Autodesk Inventor part; units mm, degrees
ref_plane "YZ Plane" through (0, 0, 0) normal (1, 0, 0) x (0, 1, 0)
ref_plane "XZ Plane" through (0, 0, 0) normal (0, 1, 0) x (-1, 0, 0)
ref_plane "XY Plane" through (0, 0, 0) normal (0, 0, 1) x (1, 0, 0)
sketch "Sketch1" plane through (0, 0, 0) normal (0, 0, 1) x (1, 0, 0)
  spline S0 degree 3 poles (12.7758, 13.7437) (13.4536, 14.296) (14.1651, 14.793) (16.9373, 16.4418) (19.2243, 17.2436) (24.5957, 17.9791) (27.7237, 17.5963) (32.8694, 15.5351) (34.9647, 14.1297) (38.6283, 10.3594) (40.0896, 7.8966) (41.4354, 3.545) (41.7033, 1.7728) (41.7033, 0) (41.7033, -1.7729) (41.4354, -3.5451) (40.0895, -7.897) (38.6278, -10.3602) (34.9655, -14.1286) (32.8727, -15.5328) (27.7225, -17.598) (24.5861, -17.9808) (19.2198, -17.2406) (16.945, -16.4433) (14.1759, -14.8006) (13.4587, -14.3002) (12.7758, -13.7437) knots 0.047577 0.047577 0.047577 0.047577 0.308418 0.308418 1.015437 1.015437 1.927825 1.927825 2.666741 2.666741 3.497446 3.497446 4.02653 4.02653 4.02653 4.555615 4.555615 5.386442 5.386442 6.124601 6.124601 7.039356 7.039356 7.74266 7.74266 8.00548 8.00548 8.00548 8.00548 weights 1 1 1 1 1 1 1 1 1 1 1 1 1 1 1 1 1 1 1 1 1 1 1 1 1 1 1
  spline S1 degree 3 poles (12.7758, -13.7437) (12.3265, -13.3776) (11.8219, -13.0794) (10.6568, -12.62) (9.9847, -12.4901) (9.3118, -12.4901) knots 0 0 0 0 0.462707 0.462707 1 1 1 1 weights 1 1 1 1 1 1
  line L0 (9.3118, -12.4901) -> (-31.0253, -12.4901)
  spline S2 degree 3 poles (9.3118, 12.4901) (9.7991, 12.4901) (10.2862, 12.5578) (11.492, 12.896) (12.1826, 13.2604) (12.7758, 13.7437) knots 0 0 0 0 0.389114 0.389114 1 1 1 1 weights 1 1 1 1 1 1
  line L1 (0, 0) -> (-42.2873, 0) construction
  line L2 (9.3118, 12.4901) -> (-31.0253, 12.4901)
  arc A0 (-31.0253, 12.4901) -> (-31.0253, -12.4901) centre (-31.0253, 0) ccw
extrude "Extrusion1" add sketch "Sketch1" along normal blind 2.5
chamfer "Chamfer1" distance 2 angle 50 6 edges at (41.7033, 0, 2.5) (11.1518, -12.8172, 2.5) (-10.8568, -12.4901, 2.5) (-43.5155, 0, 2.5) (-10.8568, 12.4901, 2.5) (11.1517, 12.8172, 2.5) measured on face at (-4.1339, -4.1634, 2.5)
sketch "Sketch6" plane through (0, 0, 2.5) normal (0, 0, 1) x (1, 0, 0)
  line L0 (-9.5253, -2.5425) -> (-15.3564, -2.5425) construction
  line L1 (-15.3564, -2.5425) -> (-15.3564, 2.5425) construction
  line L2 (-15.3564, 2.5425) -> (-9.5253, 2.5425) construction
  line L3 (-9.5253, 2.5425) -> (-9.5253, -2.5425) construction
  point P0 (0, 0)
  point P1 (-6.2263, 0)
decal "Decal1"
ref_plane "Work Plane1" through (0, 0, 0) normal (0.2164396, 0, 0.976296) x (0, 1, 0)
sketch "Sketch7" plane through (0, 0, 0) normal (0.2164396, 0, 0.976296) x (0, 1, 0)
  point P0 (0, 0)
ref_plane "Work Plane2" through (0, 0, 0) normal (0.2164396, 0, 0.976296) x (0, 1, 0)
properties part number "gornji shiny dio"
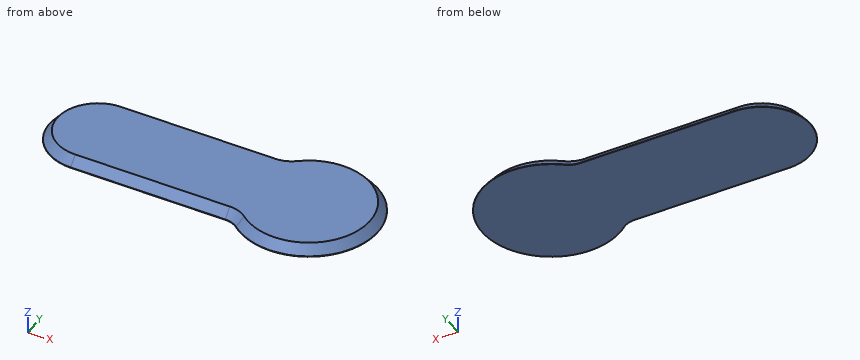
For this review, take the finished solid that the model builds, in its own axes (mm). Round coordinates to 2 decimals unless told otherwise and drop trailing zeros. Loops run counter-clockwise (first coordinate to the right, second up) from the corner with the lowest first, then second, coordinate; pieces in that order, holes last.
(1) Wall thickness on line 1 along Y through (x, z) = (-10, 1.3); line 2 along Y through (x, z) = (-6, 1.55); line 3 along X through (y, z) = (-8.5, 2.35): over which ranges is each line inside the solid? List them lowest first.
Returned:
line 1: y = -11.5 to 11.5
line 2: y = -11.29 to 11.29
line 3: x = -37.39 to 37.35
(2) We need section A-A (x = -10). Give the boundary of the cut face in (y, z), plus the area to 3 significant figures.
Returned:
outline: (-12.49, 0) - (12.49, 0) - (12.49, 0.12) - (10.49, 2.5) - (-10.49, 2.5) - (-12.49, 0.12) - close
area: 57.7 mm2
(3) Clearance check with flat-ended pins moving along their axes: P1, Ø1, axis at y = -11, z = 1.5, coming from the +X side; P2, Ø1, axis at y = 8, z = 1.5, coming from the -X side. State where each tip first meets the part, or that it passes through.
Returned:
P1: stops at x = 37.06
P2: stops at x = -39.79
